from build123d import *

# Parameters (mm, degrees)
SKETCH1_W                    = 533.4
SKETCH1_H                    = 596.9
BOSS_EXTRUDE1_DEPTH          = 3.175
CUT_EXTRUDE1_DEPTH           = 401.264129201
F_0_257_DIAMETER_SLOT1_DEPTH = 3.175
SKETCH8_W                    = 38.1
SKETCH8_H                    = 44.45
CUT_EXTRUDE2_DEPTH           = 401.264129201
FILLET1_R                    = 3.175


# Read off the part's stored shape, not the designer's step: F (0.257) Diameter Slot1
with BuildPart() as part:
    # Sketch1 → Boss-Extrude1 (new body)
    with BuildSketch(Plane(origin=(0, 0, 0), x_dir=(1, 0, 0), z_dir=(0, 1, 0))):
        Rectangle(SKETCH1_W, SKETCH1_H)
    extrude(amount=BOSS_EXTRUDE1_DEPTH)

    # Sketch5 → Cut-Extrude1 (cut, through all)
    with BuildSketch(Plane.XZ):
        with BuildLine():
            Line((244.385805934, -101.878160113), (244.385805934, -107.950617892))
            ThreePointArc((244.385805934, -107.950617892), (247.65, -111.213899987), (250.913605875, -107.950029643))
            Line((250.913605875, -107.950029643), (250.913605875, -101.878279337))
            ThreePointArc((250.913605875, -101.878279337), (247.65, -85.775799987), (244.385805934, -101.878160113))
        make_face()
        with BuildLine():
            Line((250.9139, 177.521780271), (250.9139, 171.450000343))
            ThreePointArc((250.9139, 171.450000343), (247.65, 168.1861), (244.3861, 171.450000343))
            Line((244.3861, 171.450000343), (244.3861, 177.521780271))
            ThreePointArc((244.3861, 177.521780271), (247.65, 193.6242), (250.9139, 177.521780271))
        make_face()
        with BuildLine():
            Line((-244.3861, 177.521780271), (-244.3861, 171.450000343))
            ThreePointArc((-244.3861, 171.450000343), (-247.65, 168.1861), (-250.9139, 171.450000343))
            Line((-250.9139, 171.450000343), (-250.9139, 177.521780271))
            ThreePointArc((-250.9139, 177.521780271), (-247.65, 193.6242), (-244.3861, 177.521780271))
        make_face()
        with BuildLine():
            Line((-250.913605875, -101.878279337), (-250.913605875, -107.950029643))
            ThreePointArc((-250.913605875, -107.950029643), (-247.65, -111.213899987), (-244.385805934, -107.950617892))
            Line((-244.385805934, -107.950617892), (-244.385805934, -101.878160113))
            ThreePointArc((-244.385805934, -101.878160113), (-247.65, -85.775799987), (-250.913605875, -101.878279337))
        make_face()
    extrude(amount=-CUT_EXTRUDE1_DEPTH, mode=Mode.SUBTRACT)

    # F (0.257) Diameter Slot1 outline → F (0.257) Diameter Slot1 (cut)
    with BuildSketch(Plane(origin=(0, 0, 0), x_dir=(1, 0, 0), z_dir=(0, 1, 0))):
        with BuildLine():
            ThreePointArc((252.3236, -174.7139), (255.5875, -171.45), (252.3236, -168.1861))
            Line((252.3236, -168.1861), (247.65, -168.1861))
            ThreePointArc((247.65, -168.1861), (249.957925944, -169.142074298), (250.9139, -171.450000343))
            Line((250.9139, -171.450000343), (250.9139, -174.7139))
            Line((250.9139, -174.7139), (252.3236, -174.7139))
        make_face()
        with BuildLine():
            ThreePointArc((244.3861, -171.450000343), (245.342074056, -169.142074298), (247.65, -168.1861))
            Line((247.65, -168.1861), (242.9764, -168.1861))
            ThreePointArc((242.9764, -168.1861), (239.7125, -171.45), (242.9764, -174.7139))
            Line((242.9764, -174.7139), (244.3861, -174.7139))
            Line((244.3861, -174.7139), (244.3861, -171.450000343))
        make_face()
        with BuildLine():
            ThreePointArc((-242.9764, -174.7139), (-239.7125, -171.45), (-242.9764, -168.1861))
            Line((-242.9764, -168.1861), (-247.65, -168.1861))
            ThreePointArc((-247.65, -168.1861), (-245.342074056, -169.142074298), (-244.3861, -171.450000343))
            Line((-244.3861, -171.450000343), (-244.3861, -174.7139))
            Line((-244.3861, -174.7139), (-242.9764, -174.7139))
        make_face()
        with BuildLine():
            ThreePointArc((-250.9139, -171.450000343), (-249.957925944, -169.142074298), (-247.65, -168.1861))
            Line((-247.65, -168.1861), (-252.3236, -168.1861))
            ThreePointArc((-252.3236, -168.1861), (-255.5875, -171.45), (-252.3236, -174.7139))
            Line((-252.3236, -174.7139), (-250.9139, -174.7139))
            Line((-250.9139, -174.7139), (-250.9139, -171.450000343))
        make_face()
        with BuildLine():
            ThreePointArc((252.323305875, 104.6861), (255.587205875, 107.95), (252.323305875, 111.2139))
            Line((252.323305875, 111.2139), (247.649705875, 111.2139))
            ThreePointArc((247.649705875, 111.2139), (249.957621218, 110.257936304), (250.913605875, 107.950029643))
            Line((250.913605875, 107.950029643), (250.913605875, 104.6861))
            Line((250.913605875, 104.6861), (252.323305875, 104.6861))
        make_face()
        with BuildLine():
            ThreePointArc((244.385805934, 107.950617892), (245.34199852, 110.258144271), (247.649705875, 111.2139))
            Line((247.649705875, 111.2139), (242.976105875, 111.2139))
            ThreePointArc((242.976105875, 111.2139), (239.712205875, 107.95), (242.976105875, 104.6861))
            Line((242.976105875, 104.6861), (244.385805934, 104.6861))
            Line((244.385805934, 104.6861), (244.385805934, 107.950617892))
        make_face()
        with BuildLine():
            ThreePointArc((-242.976105875, 104.6861), (-239.712205875, 107.95), (-242.976105875, 111.2139))
            Line((-242.976105875, 111.2139), (-247.649705876, 111.2139))
            ThreePointArc((-247.649705876, 111.2139), (-245.341998521, 110.258144271), (-244.385805934, 107.950617892))
            Line((-244.385805934, 107.950617892), (-244.385805934, 104.6861))
            Line((-244.385805934, 104.6861), (-242.976105875, 104.6861))
        make_face()
        with BuildLine():
            ThreePointArc((-250.913605875, 107.950029643), (-249.957621218, 110.257936303), (-247.649705876, 111.2139))
            Line((-247.649705876, 111.2139), (-252.323305875, 111.2139))
            ThreePointArc((-252.323305875, 111.2139), (-255.587205875, 107.95), (-252.323305875, 104.6861))
            Line((-252.323305875, 104.6861), (-250.913605875, 104.6861))
            Line((-250.913605875, 104.6861), (-250.913605875, 107.950029643))
        make_face()
    extrude(amount=F_0_257_DIAMETER_SLOT1_DEPTH, mode=Mode.SUBTRACT)

    # Sketch8 → Cut-Extrude2 (cut, through all)
    with BuildSketch(Plane.XZ):
        with Locations((-247.65, 31.75)):
            Rectangle(SKETCH8_W, SKETCH8_H)
        with Locations((247.65, 31.75)):
            Rectangle(SKETCH8_W, SKETCH8_H)
    extrude(amount=-CUT_EXTRUDE2_DEPTH, mode=Mode.SUBTRACT)

    # Fillet1
    fillet1_edges = [part.edges().sort_by_distance(p)[0] for p in [
        (-228.6, 1.5875, 53.975),
        (-228.6, 1.5875, 9.525),
        (228.6, 1.5875, 9.525),
        (228.6, 1.5875, 53.975),
    ]]
    fillet(fillet1_edges, radius=FILLET1_R)


solid = part.part
Work out the finished part from the listing and answer in its coordinate system (mm). Round coordinates to 2 decimals unless told otherwise and drop trailing zeros. One line per item, written item: value.
Q1. This flat-tipped pin is pushed along its axis until it touches: pin 1 Ø2 at (x, z) = (-26.5, 216.5) entering from -Y. Where does it stop, or does it pass through?
Check values:
pin 1: y = 0
Q2. The mould has two halves that part along X. Classify faces 1 (the cylindrical face through (247.33, 1.57, 193.62)), 2 (the flat face through (-4, 3.175, -4)): +X half, -X half, draft (parallel to the pull), parting line (faces both ways), or undercut.
Check values:
face 1: undercut
face 2: draft
Q3. Straight lines are drawn through the part: probe 1 along Z at (x, y) = (247.65, 2.35) (3 decimals); probe 2 along Z at (x, y) = (-233, 0.2) (3 decimals). For each, find the intervals that lie inside material, in ascending order.
Check values:
probe 1: -298.45 to -111.214, -85.776 to 9.525, 53.975 to 168.186, 193.624 to 298.45
probe 2: -298.45 to 9.525, 53.975 to 298.45
